from build123d import *

# Parameters (mm, degrees)
SKETCH1_W           = 40
SKETCH1_H           = 40
BOSS_EXTRUDE1_DEPTH = 20
SKETCH3_R           = 10
BOSS_EXTRUDE2_DEPTH = 3


with BuildPart() as part:
    # Sketch1 → Boss-Extrude1 (new body)
    with BuildSketch(Plane(origin=(0, 0, 0), x_dir=(1, 0, 0), z_dir=(0, 1, 0))):
        with Locations((20, 20)):
            Rectangle(SKETCH1_W, SKETCH1_H)
    extrude(amount=BOSS_EXTRUDE1_DEPTH)

    # Sketch3 → Boss-Extrude2 (add)
    with BuildSketch(Plane.XY):
        with Locations((30, 10)):
            Circle(SKETCH3_R)
    extrude(amount=BOSS_EXTRUDE2_DEPTH)


solid = part.part
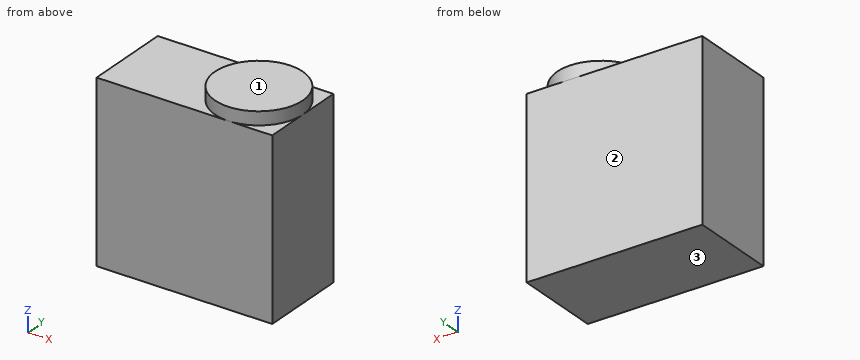
Input: part model. Units: mm. Frame: model coordinates. Face numbers are marked on the shaded views. Coordinates: 2 decimals unless noted, no trailing zeros. Write each loop counter-clockwise with the first axis right and the second up, starting at its lowest first coordinate (ties: lowest second). Pieces come first, ordered by that corner, then holes. Notation, with made-up numbers: M -23.5,67 L -6.5,67 A30 ccw -6.5,91 Z; hole C 72.5,18 d9. An arc over 180 degrees is marked long. Answer as a JSON object with one key per item and string values. Group by question number.
(1) Mould query, pull axis Z, two halves, no side actions, for the marked faces 1, 2 and 3. Classes: pulls with the +Z half, pulls with the -Z half, needs draft (parallel to the pull), parting line crosses it, or undercut.
(2) Ray query, line 1 along Z through (x, y) = (21.5, 19.25); line 2 along Y through (x, z) = (24, 0.5). Return the intervals inside material, ascending. Write a range as [from, to].
(3) Section A-A on y = 4. Output: boundary loops of the cut face in (x, z), plus the area to 3 significant figures.
(4) Contact query for flat-ended pins moving along their axis: P1, Ø8, axis at x = 11.5, z = -3.5, coming from the -Y side; P2, Ø6, axis at x = 12, y = 10.5, coming from the +Z side. Output: stop coordinate, or through.
(5) Section B-B on x = 23.5. Output: boundary loops of the cut face in (y, z).
Result set:
{
 "1": {"face 1": "pulls with the +Z half", "face 2": "needs draft", "face 3": "pulls with the -Z half"},
 "2": {"line 1": "z = [-40, 0]", "line 2": "y = [2, 18]"},
 "3": {"outline": "M 0,-40 L 40,-40 L 40,0 L 38,0 L 38,3 L 22,3 L 22,0 L 0,0 Z", "area": "1,650 mm2"},
 "4": {"P1": "stops at y = 0", "P2": "stops at z = 0"},
 "5": {"outline": "M 0,-40 L 20,-40 L 20,0 L 17.6,0 L 17.6,3 L 2.4,3 L 2.4,0 L 0,0 Z"}
}
